CAD build for the part. Positions are in the model's coordinates, mm. Round coordinates to 2 decimals unless told otherwise and drop trailing zeros. Loops run counter-clockwise (first coordinate to the right, second up) from the corner with the lowest first, then second, coordinate; pieces in that order, holes last.
```python
from build123d import *

# Parameters (mm, degrees)
ESQUISSE1_W        = 54
ESQUISSE1_H        = 60
ESQUISSE1_R        = 2
ESQUISSE1_W_2      = 46
BOSS_EXTRU_1_DEPTH = 17


with BuildPart() as part:
    # Esquisse1 → Boss.-Extru.1 (new body)
    # profile 1 of 3: a face of its own
    with BuildSketch(Plane.XY):
        with Locations((27, -30)):
            Rectangle(ESQUISSE1_W, ESQUISSE1_H)
        with Locations((27, -5)):
            Circle(ESQUISSE1_R, mode=Mode.SUBTRACT)
        with Locations((27, -30)):
            Circle(ESQUISSE1_R, mode=Mode.SUBTRACT)
        with Locations((27, -55)):
            Circle(ESQUISSE1_R, mode=Mode.SUBTRACT)
    # profile 2 of 3: a face of its own
    with BuildSketch(Plane.XY):
        with Locations((77, -30)):
            Rectangle(ESQUISSE1_W_2, ESQUISSE1_H)
    # profile 3 of 3: a face of its own
    with BuildSketch(Plane.XY):
        with Locations((127, -30)):
            Rectangle(ESQUISSE1_W, ESQUISSE1_H)
    extrude(amount=BOSS_EXTRU_1_DEPTH)


solid = part.part
```
Item 1: Two-plate mould, pull along Y, no slides. Class faces 1 (the cylindrical face through (27.923, -31.774, 8.381)), 2 (the flat face through (76, 0, 8)), 3 (the cylindrical face through (28.075, -53.314, 8.381)), 4 (the flat face through (76, -60, 8)): released by +Y, released by -Y, zero draft, split by the parting line, or undercut.
Answers follow:
face 1: undercut
face 2: released by +Y
face 3: undercut
face 4: released by -Y
Item 2: Probe line 1 (Y direction, x = 27, z = 13); line 2 (X direction, y = -56, z = 7.5). List the from-to ranges inside material, lowest first.
Answers follow:
line 1: y = -60 to -57, -53 to -32, -28 to -7, -3 to 0
line 2: x = 0 to 25.27, 28.73 to 154
Item 3: Cut at B-B, the plane x = 27. Give the cut face in (y, z), plus the area to 3 significant figures.
Answers follow:
outline: (-60, 0) - (-57, 0) - (-57, 17) - (-60, 17) - close; (-53, 0) - (-32, 0) - (-32, 17) - (-53, 17) - close; (-28, 0) - (-7, 0) - (-7, 17) - (-28, 17) - close; (-3, 0) - (0, 0) - (0, 17) - (-3, 17) - close
area: 816 mm2
Item 4: Cut at A-A, the plane y = -5. Give the cut face in (x, z), plus the area to 3 significant figures.
Answers follow:
outline: (0, 0) - (25, 0) - (25, 17) - (0, 17) - close; (29, 0) - (154, 0) - (154, 17) - (29, 17) - close
area: 2,550 mm2
